For this review, take the finished solid that the model builds, in its own axes (mm). Face numbers are marked on the shaded views. A direction names the side the tool comes from. Round coordinates to 2 decimals unless told otherwise and drop trailing zeros. Write each loop counter-clockwise with the first axis right and the second up, starting at its lowest first coordinate (ties: lowest second). Pieces come first, ordered by that corner, then holes. Notation, with made-up numbers: (58.25, 0.5) -> (98.25, 0.5) arc R24 cw to (98.25, 10.5) -> close; hole circle Ø8 at (48.25, 86). An arc over 180 degrees is marked (long way). Write each question's results on one line, items separated by ' | '. Start each with the question number.
Item 1: The part is to be moulded in two halves that separate along X. For the marked faces 6, 7 and 8, say which applies: +X half, -X half, draft (parallel to the pull), parting line (faces both ways), or undercut.
Item 2: Add section A-A (z = -22). State the section outline as (x, y) points.
Item 3: To check wall thickness, follow line 1 along Y through (x, z) = (0, -2.95); line 2 along Z through (x, y) = (-1.5, 4.25); line 3 along Z through (x, y) = (-2.5, 2.5). State the ranges of each line that lie inside material, in increasing order.
Item 4: Add section B-B (x = 0). State the section outline as (y, z) points, plus the area to 3 significant figures.
Item 5: Add section D-D (z = -11). State the section outline as (x, y) points, plus the area to 3 significant figures.
Item 6: Tool access review of the marked faces 1, 2, 3, 4 and 5: name each direction out of +Z, -Z, +X, -X, +Y, -Y from which nothing blocks a thin tool from reaching the whole face with its end or side.
Item 7: Add section C-C (y = 0). State the section outline as (x, z) points.
Item 8: Clearance check with flat-ended pins moving along their axes: pin 1 (1.4 mm diameter, centred on y = 0.5, z = -21.5, fed in from +X); pin 2 (3 mm diameter, centred on x = 1, y = 0.5, fed in from -Z); pin 3 (6 mm diameter, centred on x = 4, z = -6.5, fed in from -Y). State where each tip first meets the part, or that it passes through.
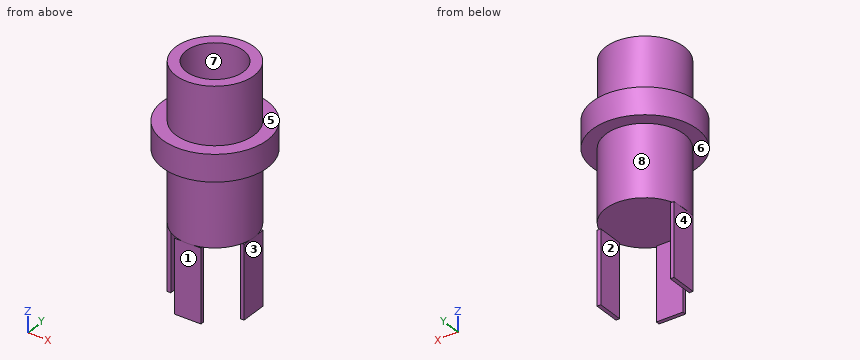
from build123d import *

# Parameters (mm, degrees)
SKETCH1_R           = 4.1
SKETCH1_R_2         = 3
BOSS_EXTRUDE1_DEPTH = 6
SKETCH2_R           = 5.5
BOSS_EXTRUDE2_DEPTH = 2.8
SKETCH3_R           = 4.1
BOSS_EXTRUDE3_DEPTH = 7.5
SKETCH4_W           = 0.4
SKETCH4_H           = 2.8
SKETCH4_W_2         = 2.8
SKETCH4_H_2         = 0.4
EXTRUDE_THIN1_DEPTH = 7.65


with BuildPart() as part:
    # Sketch1 → Boss-Extrude1 (new body)
    with BuildSketch(Plane.XY):
        Circle(SKETCH1_R)
        Circle(SKETCH1_R_2, mode=Mode.SUBTRACT)
    extrude(amount=-BOSS_EXTRUDE1_DEPTH)

    # Sketch2 → Boss-Extrude2 (add)
    with BuildSketch(Plane(origin=(0, 0, -6), x_dir=(-1, 0, 0), z_dir=(0, 0, -1))):
        Circle(SKETCH2_R)
    extrude(amount=BOSS_EXTRUDE2_DEPTH)

    # Sketch3 → Boss-Extrude3 (add)
    with BuildSketch(Plane(origin=(0, 0, -8.8), x_dir=(-1, 0, 0), z_dir=(0, 0, -1))):
        Circle(SKETCH3_R)
    extrude(amount=BOSS_EXTRUDE3_DEPTH)

    # Sketch4 → Extrude-Thin1 (add)
    with BuildSketch(Plane(origin=(0, 0, -16.3), x_dir=(-1, 0, 0), z_dir=(0, 0, -1))):
        with Locations((-3.853569774, 0)):
            Rectangle(SKETCH4_W, SKETCH4_H)
        with Locations((0, -3.853569774)):
            Rectangle(SKETCH4_W_2, SKETCH4_H_2)
        with Locations((3.853569774, 0)):
            Rectangle(SKETCH4_W, SKETCH4_H)
    extrude(amount=EXTRUDE_THIN1_DEPTH)


solid = part.part
Responses:
1) face 6: draft | face 7: undercut | face 8: parting line
2) outline: (-4.05, -1.4) -> (-3.65, -1.4) -> (-3.65, 1.4) -> (-4.05, 1.4) -> close; (-1.4, -4.05) -> (1.4, -4.05) -> (1.4, -3.65) -> (-1.4, -3.65) -> close; (3.65, -1.4) -> (4.05, -1.4) -> (4.05, 1.4) -> (3.65, 1.4) -> close
3) line 1: y = -4.1 to -3, 3 to 4.1 | line 2: z = -8.8 to -6 | line 3: z = -16.3 to 0
4) outline: (-5.5, -8.8) -> (-4.1, -8.8) -> (-4.1, -16.3) -> (-4.05, -16.3) -> (-4.05, -23.95) -> (-3.65, -23.95) -> (-3.65, -16.3) -> (4.1, -16.3) -> (4.1, -8.8) -> (5.5, -8.8) -> (5.5, -6) -> (4.1, -6) -> (4.1, 0) -> (3, 0) -> (3, -6) -> (-3, -6) -> (-3, 0) -> (-4.1, 0) -> (-4.1, -6) -> (-5.5, -6) -> close | area: 109 mm^2
5) outline: circle Ø8.2 at (0, 0) | area: 52.8 mm^2
6) face 1: -Z, +X, -X, -Y | face 2: -Z, +Y, -Y | face 3: -Z, +X, +Y, -Y | face 4: -Z, -X, +Y, -Y | face 5: +Z
7) outline: (-5.5, -8.8) -> (-4.1, -8.8) -> (-4.1, -16.3) -> (-4.05, -16.3) -> (-4.05, -23.95) -> (-3.65, -23.95) -> (-3.65, -16.3) -> (3.65, -16.3) -> (3.65, -23.95) -> (4.05, -23.95) -> (4.05, -16.3) -> (4.1, -16.3) -> (4.1, -8.8) -> (5.5, -8.8) -> (5.5, -6) -> (4.1, -6) -> (4.1, 0) -> (3, 0) -> (3, -6) -> (-3, -6) -> (-3, 0) -> (-4.1, 0) -> (-4.1, -6) -> (-5.5, -6) -> close
8) pin 1: stops at x = 4.05 | pin 2: stops at z = -16.3 | pin 3: stops at y = -5.41
